Work out the finished part from the listing and answer in its coordinate system (mm). Round coordinates to 2 decimals unless told otherwise and drop trailing zeros. Loops run counter-clockwise (first coordinate to the right, second up) from the corner with the lowest first, then second, coordinate; pieces in that order, holes last.
Autodesk Inventor part; units mm, degrees
ref_plane "YZ Plane" through (0, 0, 0) normal (1, 0, 0) x (0, 1, 0)
ref_plane "XZ Plane" through (0, 0, 0) normal (0, 1, 0) x (-1, 0, 0)
ref_plane "XY Plane" through (0, 0, 0) normal (0, 0, 1) x (1, 0, 0)
sketch "Sketch1" plane through (0, 0, 0) normal (1, 0, 0) x (0, 1, 0)
  line L0 (-17.5, 57.5) -> (17.5, 57.5)
  line L1 (17.5, 57.5) -> (17.5, -57.5)
  line L2 (17.5, -57.5) -> (-17.5, -57.5)
  line L3 (-17.5, -57.5) -> (-17.5, 57.5)
  line L4 (-17.5, 57.5) -> (17.5, -57.5) construction
  line L5 (17.5, 57.5) -> (-17.5, -57.5) construction
  point P0 (0, 0)
  dimension "d0" = 35
  dimension "d1" = 115
extrude "Extrusion1" add sketch "Sketch1" along normal blind 3
sketch "Sketch2" plane through (3, 0, 0) normal (1, 0, 0) x (0, 0, -1)
  line L0 (-57.5, -17.5) -> (57.5, -17.5)
  line L1 (-42.5, -17.5) -> (-22.5, -17.5)
  line L2 (-22.5, -17.5) -> (-22.5, -20.5)
  line L3 (-22.5, -20.5) -> (-42.5, -20.5)
  line L4 (-42.5, -20.5) -> (-42.5, -17.5)
  line L5 (-57.5, 17.5) -> (-57.5, -17.5)
  line L6 (-2.5, -17.5) -> (17.5, -17.5)
  line L7 (17.5, -17.5) -> (17.5, -20.5)
  line L8 (17.5, -20.5) -> (-2.5, -20.5)
  line L9 (-2.5, -20.5) -> (-2.5, -17.5)
  line L10 (37.5, -17.5) -> (57.5, -17.5)
  line L11 (57.5, -17.5) -> (57.5, -20.5)
  line L12 (57.5, -20.5) -> (37.5, -20.5)
  line L13 (37.5, -20.5) -> (37.5, -17.5)
  point P0 (0, 0)
  dimension "d4" = 20
  dimension "d5" = 3
  dimension "d6" = 15
  dimension "d7" = 20
  dimension "d8" = 3
  dimension "d9" = 20
  dimension "d10" = 20
  dimension "d11" = 3
  dimension "d12" = 20
extrude "Extrusion2" add sketch "Sketch2" against normal blind 3
sketch "Sketch3" plane through (3, 0, 0) normal (1, 0, 0) x (0, 0, -1)
  line L0 (-57.5, -17.5) -> (-57.5, 17.5)
  line L1 (-57.5, 10) -> (-60.5, 10)
  line L2 (-60.5, 10) -> (-60.5, -10)
  line L3 (-60.5, -10) -> (-57.5, -10)
  line L4 (-57.5, -10) -> (-57.5, 10)
  point P0 (0, 0)
  point P1 (-60.5, 0)
  dimension "d15" = 3
  dimension "d16" = 20
extrude "Extrusion3" add sketch "Sketch3" against normal blind 3
sketch "Sketch4" plane through (3, 0, 0) normal (1, 0, 0) x (0, 0, -1)
  line L0 (-26.5, -7.5) -> (-14.5, -7.5)
  line L1 (-14.5, -7.5) -> (-14.5, 2.5)
  line L2 (-14.5, 2.5) -> (-26.5, 2.5)
  line L3 (-26.5, 2.5) -> (-26.5, -7.5)
  line L4 (-26.5, -7.5) -> (-14.5, 2.5) construction
  line L5 (-14.5, -7.5) -> (-26.5, 2.5) construction
  circle A0 centre (-20.5, -2.5) radius 2
  point P0 (0, 0)
  point P1 (-20.5, -2.5)
  dimension "d19" = 12
  dimension "d20" = 10
extrude "Extrusion4" cut sketch "Sketch4" against normal blind 3 contours L3 L2 L1 L0 | A0
sketch "Sketch5" plane through (3, 0, 0) normal (1, 0, 0) x (0, 0, -1)
  line L0 (-57.5, 17.5) -> (57.5, 17.5)
  line L1 (22.5, 17.5) -> (25.5, 17.5)
  line L2 (25.5, 17.5) -> (25.5, 2.5)
  line L3 (25.5, 2.5) -> (22.5, 2.5)
  line L4 (22.5, 2.5) -> (22.5, 17.5)
  line L5 (-57.5, 17.5) -> (-57.5, 10)
  point P0 (0, 0)
  dimension "d23" = 3
  dimension "d24" = 15
  dimension "d25" = 80
extrude "Extrusion5" cut sketch "Sketch5" against normal blind 3
sketch "Sketch6" plane through (0, 0, 0) normal (-1, 0, 0) x (0, 0, 1)
  line L0 (-22.5, 17.5) -> (57.5, 17.5)
  line L1 (47.5, 17.5) -> (37.5, 17.5)
  line L2 (37.5, 17.5) -> (37.5, 20.5)
  line L3 (37.5, 20.5) -> (47.5, 20.5)
  line L4 (47.5, 20.5) -> (47.5, 17.5)
  line L5 (57.5, 10) -> (57.5, 17.5)
  line L6 (-2.5, 17.5) -> (17.5, 17.5)
  line L7 (17.5, 17.5) -> (17.5, 20.5)
  line L8 (17.5, 20.5) -> (-2.5, 20.5)
  line L9 (-2.5, 20.5) -> (-2.5, 17.5)
  line L10 (-25.5, 17.5) -> (-57.5, 17.5)
  line L11 (-37.5, 17.5) -> (-47.5, 17.5)
  line L12 (-47.5, 17.5) -> (-47.5, 20.5)
  line L13 (-47.5, 20.5) -> (-37.5, 20.5)
  line L14 (-37.5, 20.5) -> (-37.5, 17.5)
  point P0 (0, 0)
  dimension "d28" = 10
  dimension "d29" = 3
  dimension "d30" = 10
  dimension "d31" = 20
  dimension "d32" = 3
  dimension "d33" = 20
  dimension "d34" = 10
  dimension "d35" = 3
  dimension "d36" = 35
extrude "Extrusion6" add sketch "Sketch6" against normal blind 3
properties part number "Motor support plate"
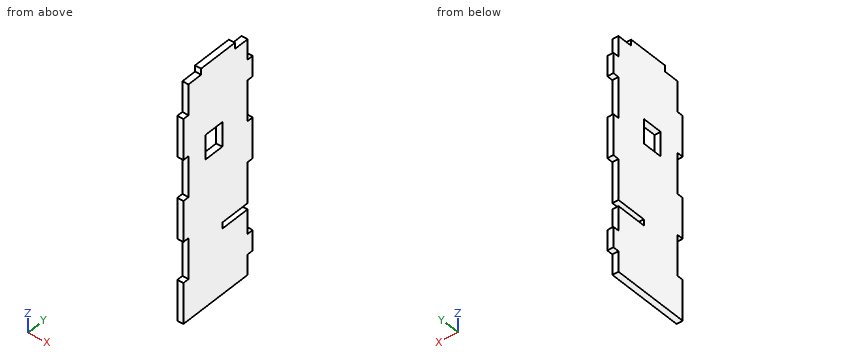
Item 1: Section C-C, the plane y = -15.5 is taken. Give the vertices of the cut face in (x, z), plus the area to 3 significant figures.
Item 2: Section D-D, the plane z = 4 is taken. Give the vertices of the cut face in (x, y).
Item 3: Straight lines are drawn through the part: line 1 (Z direction, x = 2.65, y = 13); line 2 (Z direction, x = 2.55, y = 9.5); line 3 (Z direction, x = 0.85, y = -17). For each, find the intervals that lie inside material, in ascending order.
Item 4: Section B-B, the plane z = 16.5 is taken. Give the vertices of the cut face in (x, y).
Item 5: Section A-A, the plane y = 13 is taken. Give the vertices of the cut face in (x, z).
Item 6: Each of these flat-tipped pins is pushed along its axis until it touches: P1, Ø1.5, axis at x = 2, z = 58.5, coming from the -Y side; P2, Ø0.9, axis at x = 1.5, z = -24.5, coming from the +Y side; P3, Ø1.5, axis at x = 1, z = 19, coming from the +Y side. Where does it stop, or does it pass through?
Answer below:
1. outline: (0, -57.5) - (3, -57.5) - (3, 57.5) - (0, 57.5) - close
1. area: 345 mm2
2. outline: (0, -17.5) - (3, -17.5) - (3, 20.5) - (0, 20.5) - close
3. line 1: z = -57.5 to -25.5, -22.5 to 57.5
3. line 2: z = -57.5 to -25.5, -22.5 to 60.5
3. line 3: z = -57.5 to 57.5
4. outline: (0, -17.5) - (3, -17.5) - (3, -7.5) - (0, -7.5) - close; (0, 2.5) - (3, 2.5) - (3, 20.5) - (0, 20.5) - close
5. outline: (0, -57.5) - (3, -57.5) - (3, -25.5) - (0, -25.5) - close; (0, -22.5) - (3, -22.5) - (3, 57.5) - (0, 57.5) - close
6. P1: stops at y = -10
6. P2: stops at y = 2.5
6. P3: stops at y = 17.5
